Read the model definition and answer for the solid it produces. Units are mm, in the model's axes. Face numbers are marked on the shaded views. A direction names the side the tool comes from. Give positions to 0.01 mm unless a question says otherwise; leave off trailing zeros. Order: outer loops, then holes, each group sorted by start corner. A loop starts at its lowest first (then second) coordinate and runs counter-clockwise, first axis right, second up. Notation, with made-up numbers: (-30, 64.25) - (15, 64.25) arc R6 cw to (15, 69.25) - close; hole circle Ø2 at (-38, 67.25). An arc over 180 degrees is marked (long way). Use a Markdown table: item, result. Add a question column.
1. Which of the six approach directions +Z, -Z, +X, -X, +Y, -Y give full straight-line access (tool end or side, diameter ignored) to the marked faces 1 and 2?
2. For a pull along Z with two mould halves and no side action, classify the marked faces 3, 4, 5 and 6 as released by +Z, released by -Z, zero draft, split by the parting line, or undercut.
3. A cutting plane is placed at A-A on x = -6. Determine the outline of the cut face in (y, z).
4. Consider L1, parallel to Y at x = 123.5, z = 138; L2, parallel to Z at x = 0, y = 279.5; L3, parallel to Z at x = -25.5, y = 268. Determine where each line is inside the solid, lowest interval first.
5. A cutting plane is placed at D-D on x = 69.5. Determine the outline of the cut face in (y, z).
6. A cutting plane is placed at C-C on y = 308. Determine the outline of the cut face in (x, z).
7. A flat-ended cylindrical pin translates along its axis: P1, Ø19, axis at x = 158, y = 221, coming from the +Z side. Find the tip coordinate at first contact, or state that the pin passes through.
8. A cutting plane is placed at B-B on z = -71.5. Determine the outline of the cut face in (x, y).
```python
from build123d import *

# Parameters (mm, degrees)
F1_W     = 381
F1_H     = 381
F1_R     = 127
F2_DEPTH = 381
F3_W     = 190.5
F3_H     = 127
F4_DEPTH = 190.5


with BuildPart() as f2:
    # F1 (on face) → F2 (new body)
    with BuildSketch(Plane.XZ):
        Rectangle(F1_W, F1_H)
        Circle(F1_R, mode=Mode.SUBTRACT)
    extrude(amount=-F2_DEPTH)

    # F3 (on face) → F4 (cut)
    with BuildSketch(Plane.XY.offset(190.5)):
        with Locations((95.25, 190.5)):
            Rectangle(F3_W, F3_H)
    extrude(amount=-F4_DEPTH, mode=Mode.SUBTRACT)


solid = f2.part
```
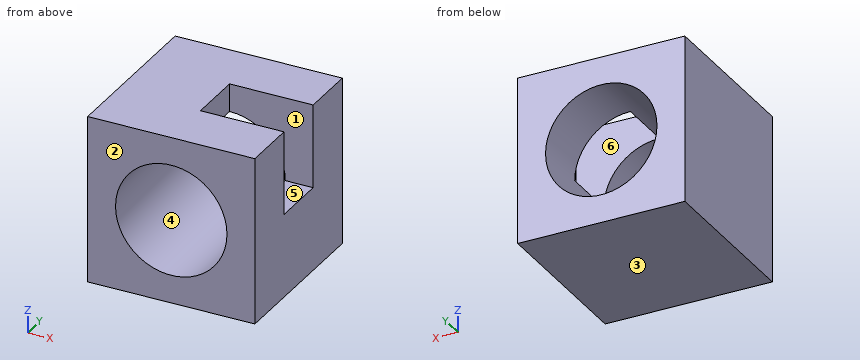
Output values:
| question | item | result |
|---|---|---|
| 1 | face 1 | +Z, +X |
| 1 | face 2 | +Z, -Z, +X, -X, -Y |
| 2 | face 3 | released by -Z |
| 2 | face 4 | undercut |
| 2 | face 5 | released by +Z |
| 2 | face 6 | zero draft |
| 3 | outline | (0, -190.5) - (381, -190.5) - (381, -126.86) - (0, -126.86) - close; (0, 126.86) - (381, 126.86) - (381, 190.5) - (0, 190.5) - close |
| 4 | L1 | 0 to 127, 254 to 381 |
| 4 | L2 | -190.5 to -127, 127 to 190.5 |
| 4 | L3 | -190.5 to -124.41, 124.41 to 190.5 |
| 5 | outline | (0, -190.5) - (381, -190.5) - (381, -106.3) - (0, -106.3) - close; (0, 106.3) - (127, 106.3) - (127, 190.5) - (0, 190.5) - close; (254, 106.3) - (381, 106.3) - (381, 190.5) - (254, 190.5) - close |
| 6 | outline | (-190.5, -190.5) - (190.5, -190.5) - (190.5, 190.5) - (-190.5, 190.5) - close; hole circle Ø254 at (0, 0) |
| 7 | P1 | z = 0 |
| 8 | outline | (-190.5, 0) - (-104.96, 0) - (-104.96, 381) - (-190.5, 381) - close; (104.96, 0) - (190.5, 0) - (190.5, 381) - (104.96, 381) - close |
